For this review, take the finished solid that the model builds, in its own axes (mm). Face numbers are marked on the shaded views. A direction names the side the tool comes from. Round coordinates to 2 decimals unless told otherwise and drop trailing zeros. Write each loop counter-clockwise with the first axis right and the second up, starting at its lowest first coordinate (ties: lowest second). Pieces come first, ordered by that corner, then holes. Notation, with made-up numbers: M -23,62 L 35,62 A3 ccw 35,66 Z; hole C 38.5,15 d4. An arc over 180 degrees is marked long. Answer in a Markdown table with one row per item.
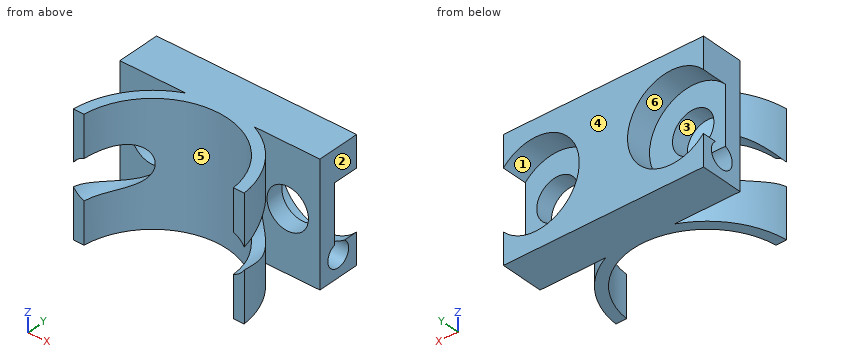
```python
from build123d import *

# Parameters (mm, degrees)
SALIENTE_EXTRUIR1_DEPTH                              = 17
TALADRO_DE_MARGEN_PARA_M31_D                         = 3.4
REFRENTADO_PARA_PERNO_CON_CABEZA_HEXAGON_D           = 5.8
REFRENTADO_PARA_PERNO_CON_CABEZA_HEXAGON_CBORE_D     = 12.24
REFRENTADO_PARA_PERNO_CON_CABEZA_HEXAGON_CBORE_DEPTH = 3.58


with BuildPart() as part:
    # Croquis1 → Saliente-Extruir1 (new body)
    with BuildSketch(Plane.XY):
        with BuildLine():
            Line((13.975508884, 11), (13.975508884, 17))
            Line((13.975508884, 17), (-14.024491116, 17))
            Line((-14.024491116, 17), (-14.024491116, 11))
            Line((-14.024491116, 11), (-4.795831523, 11))
            ThreePointArc((-4.795831523, 11), (-9.755762498, 6.987495838), (-11.958260743, 1))
            Line((-11.958260743, 1), (-10.45227248, 1))
            ThreePointArc((-10.45227248, 1), (0, 10.5), (10.45227248, 1))
            Line((10.45227248, 1), (11.958260743, 1))
            ThreePointArc((11.958260743, 1), (9.755762498, 6.987495838), (4.795831523, 11))
            Line((4.795831523, 11), (13.975508884, 11))
        make_face()
    extrude(amount=SALIENTE_EXTRUIR1_DEPTH)

    # Taladro de margen para M31 (through all)
    with Locations(Plane(origin=(13.975508884, 0, 0), x_dir=(0, 0, -1), z_dir=(1, 0, 0))):
        with Locations((-3, 14)):
            Hole(TALADRO_DE_MARGEN_PARA_M31_D / 2)

    # Refrentado para perno con cabeza hexagonal de M51 (through all)
    with Locations(Plane(origin=(0, 17, 0), x_dir=(1, 0, 0), z_dir=(0, 1, 0))):
        with Locations((9.475508884, -8.5), (-9.524491116, -8.5)):
            CounterBoreHole(REFRENTADO_PARA_PERNO_CON_CABEZA_HEXAGON_D / 2, REFRENTADO_PARA_PERNO_CON_CABEZA_HEXAGON_CBORE_D / 2, REFRENTADO_PARA_PERNO_CON_CABEZA_HEXAGON_CBORE_DEPTH)


solid = part.part
```
Q1. For probe 1 along Z at (x, y) = (12.75, 13.5); probe 2 along X at (y, z) = (2, 5); probe 3 along Y at (x, z) = (8.25, 5), list the stretches that pass through material, from the lowest coordinate up.
Found:
| item | result |
|---|---|
| probe 1 | 0 to 1.38, 13.67 to 17 |
| probe 2 | -11.83 to -10.31, 10.31 to 11.83 |
| probe 3 | 6.5 to 8.71, 11 to 13.42 |
Q2. Take a section at A-A (z = 8.5). State the section outline as (x, y) points, then the cut area to 3 significant figures.
Found:
| item | result |
|---|---|
| outline | M -14.02,11 L -12.42,11 L -12.42,13.42 L -14.02,13.42 Z; M -6.62,8.15 A10.5 cw 6.58,8.19 L 6.58,10.04 A12 ccw 4.8,11 L 6.58,11 L 6.58,13.42 L 3.36,13.42 L 3.36,17 L -3.4,17 L -3.4,13.42 L -6.62,13.42 L -6.62,11 L -4.8,11 A12 ccw -6.62,10.01 Z; M 12.38,11 L 13.98,11 L 13.98,13.42 L 12.38,13.42 Z |
| area | 78.6 mm² |
Q3. Mouldability with a two-part tool opening along X and no side actions: class the marked faces 1, 2, 3 and 4 as +X half, -X half, draft (parallel to the pull), parting line (faces both ways), or undercut.
Found:
| item | result |
|---|---|
| face 1 | undercut |
| face 2 | +X half |
| face 3 | undercut |
| face 4 | draft |
Q4. Take a section at D-D (z = 3). State the section outline as (x, y) points, then the cut area to 3 significant figures.
Found:
| item | result |
|---|---|
| outline | M -14.02,11 L -4.8,11 A12 ccw -11.96,1 L -10.45,1 A10.5 cw 10.45,1 L 11.96,1 A12 ccw 4.8,11 L 13.98,11 L 13.98,12.3 L -14.02,12.3 Z; M -14.02,15.7 L -12.21,15.7 L -12.21,17 L -14.02,17 Z; M -6.84,15.7 L 6.79,15.7 L 6.79,17 L -6.84,17 Z; M 12.16,15.7 L 13.98,15.7 L 13.98,17 L 12.16,17 Z |
| area | 102 mm² |
Q5. Take a section at B-B (x = 8.75). State the section outline as (y, z) points, then the cut area to 3 significant figures.
Found:
| item | result |
|---|---|
| outline | M 5.8,0 L 8.21,0 L 8.21,5.69 L 5.8,5.69 Z; M 5.8,11.31 L 8.21,11.31 L 8.21,17 L 5.8,17 Z; M 11,0 L 17,0 L 17,2.42 L 15.6,2.42 A1.7 cw long 13.42,4.6 L 13.42,5.69 L 11,5.69 Z; M 11,11.31 L 13.42,11.31 L 13.42,14.58 L 17,14.58 L 17,17 L 11,17 Z |
| area | 67.8 mm² |
Q6. Take a section at C-C (y = 5). State the section outline as (x, z) points, then the cut area to 3 significant figures.
Found:
| item | result |
|---|---|
| outline | M -10.91,0 L -9.23,0 L -9.23,5.61 A2.9 cw -10.91,5.95 Z; M -10.91,11.05 A2.9 cw -9.23,11.39 L -9.23,17 L -10.91,17 Z; M 9.23,0 L 10.91,0 L 10.91,5.98 A2.9 cw 9.23,5.61 Z; M 9.23,11.39 A2.9 cw 10.91,11.02 L 10.91,17 L 9.23,17 Z |
| area | 38.2 mm² |
Q7. Insertion check: P1, Ø5, axis at x = 5, z = 15, coming from the -Y side; P2, Ø3, axis at y = 7.5, z = 14, coming from the -X side; P3, Ø7.5, axis at x = -9.52, z = 8.5, coming from the +Y side; P4, Ø3.5, axis at x = 9.48, z = 8.5, coming from the +Y side. Each pin has a flat end and moves straight along its axis. Give the tip position at first contact, or say it passes through.
Found:
| item | result |
|---|---|
| P1 | y = 7.35 |
| P2 | x = -10.39 |
| P3 | y = 13.42 |
| P4 | through |
Q8. Machinability: for the marked faces 5 and 6, which of the approach directions +Z, -Z, +X, -X, +Y, -Y give a long, thin tool a straight path to every point of the face, cutting with its end or side? Answer none if there is none.
Found:
| item | result |
|---|---|
| face 5 | +Z, -Z, -Y |
| face 6 | +Y |
